Work out the finished part from the listing and answer in its coordinate system (mm). A direction names the side the tool comes from. Round coordinates to 2 decimals unless told otherwise and drop trailing zeros. Loops run counter-clockwise (first coordinate to the right, second up) from the corner with the lowest first, then second, coordinate; pieces in that order, holes last. Notation, with made-up numbers: (3.5, 77) - (12.5, 77) arc R17 cw to (12.5, 90) - close; hole circle Ø2 at (48.5, -16.5). An arc over 180 degrees is marked (long way). Return JSON: item names as keys, results as strings.
from build123d import *

# Parameters (mm, degrees)
BOSS_EXTRUDE1_DEPTH = 30
SKETCH2_R           = 2
CUT_EXTRUDE1_DEPTH  = 30
SKETCH3_W           = 10
SKETCH3_H           = 30
CUT_EXTRUDE2_DEPTH  = 6


with BuildPart() as part:
    # Sketch1 → Boss-Extrude1 (new body)
    with BuildSketch(Plane(origin=(0, 0, 0), x_dir=(0, 1, 0), z_dir=(0, 0, 1))):
        Polygon((0, 0), (-30, 0), (-30, -30), (-27, -30), (-27, -3), (0, -3), align=None)
    extrude(amount=BOSS_EXTRUDE1_DEPTH)

    # Sketch2 → Cut-Extrude1 (cut)
    with BuildSketch(Plane(origin=(0, -27, 0), x_dir=(-1, 0, 0), z_dir=(0, 1, 0))):
        with Locations(Location((-15, 15, 0), (0, 0, 90))):
            Circle(SKETCH2_R)
    extrude(amount=-CUT_EXTRUDE1_DEPTH, mode=Mode.SUBTRACT)

    # Sketch3 → Cut-Extrude2 (cut)
    with BuildSketch(Plane(origin=(0, -27, 0), x_dir=(-1, 0, 0), z_dir=(0, 1, 0))):
        with Locations((-25, 15)):
            Rectangle(SKETCH3_W, SKETCH3_H)
    extrude(amount=-CUT_EXTRUDE2_DEPTH, mode=Mode.SUBTRACT)


solid = part.part
1) Find the intervals of material crossed by L1, parallel to X at y = -27.75, z = 15; L2, parallel to X at y = -22, z = 2; L3, parallel to Y at x = 15.75, z = 23.25, in increasing order.
Verdict:
{"L1": "x = 0 to 13, 17 to 20", "L2": "x = 0 to 3", "L3": "y = -30 to -27"}
2) Flat-ended cylindrical pins translate along their axes: pin 1 (8.5 mm diameter, centred on x = 10, z = 11, fed in from +Y); pin 2 (3 mm diameter, centred on y = -8, z = 20, fed in from -X); pin 3 (13.5 mm diameter, centred on y = -18, z = 8.5, fed in from +X). Find the tip coordinate at first contact, or state that the pin passes through.
Verdict:
{"pin 1": "stops at y = -27", "pin 2": "stops at x = 0", "pin 3": "stops at x = 3"}
3) Section A-A (z = 15) is taken. Give the vertices of the cut face in (x, y), and give its area (3 significant figures).
Verdict:
{"outline": "(0, -30) - (13, -30) - (13, -27) - (3, -27) - (3, 0) - (0, 0) - close; (17, -30) - (20, -30) - (20, -27) - (17, -27) - close", "area": "129 mm2"}
4) Section B-B (x = 16.25) is taken. Give the vertices of the cut face in (y, z).
Verdict:
{"outline": "(-30, 0) - (-27, 0) - (-27, 13.44) - (-30, 13.44) - close; (-30, 16.56) - (-27, 16.56) - (-27, 30) - (-30, 30) - close"}
5) Section C-C (z = 26) is taken. Give the vertices of the cut face in (x, y).
Verdict:
{"outline": "(0, -30) - (20, -30) - (20, -27) - (3, -27) - (3, 0) - (0, 0) - close"}
6) Section D-D (y = -8.75) is taken. Give the vertices of the cut face in (x, z).
Verdict:
{"outline": "(0, 0) - (3, 0) - (3, 30) - (0, 30) - close"}
7) Determine the mould class of faces 1 (the flat face through (20, -28, 15)), 2 (the flat face through (2, 0, 15)), 3 (the cylindrical face through (17, -28, 15)) for opening direction X: pulls with the +X half, pulls with the -X half, needs draft (parallel to the pull), parting line crosses it, or undercut.
Verdict:
{"face 1": "pulls with the +X half", "face 2": "needs draft", "face 3": "undercut"}
8) A tool of negligible diameter and unlimited length cuts with its end or side. For faces 4 (the flat face through (2, -21, 30)), 5 (the flat face through (12, -27, 15)), from which of +Z, -Z, +X, -X, +Y, -Y can it reach the whole face along a straight path? Write none if from no direction.
Verdict:
{"face 4": "+Z, +X, -X, +Y, -Y", "face 5": "+Z, -Z, +X, +Y"}
